The model under review builds one solid part; all positions refer to its coordinate system, in mm. Face numbers are marked on the shaded views. A direction names the side the tool comes from. Coordinates: 2 decimals unless noted, no trailing zeros. Write each loop counter-clockwise with the first axis right and the second up, starting at its lowest first coordinate (ties: lowest second). Pieces come first, ordered by that corner, then holes.
1) Add section C-C, the plane z = -109. State the section outline as (x, y) points, then the cut area to 3 significant figures.
2) For P1, Ø6, axis at x = -9, z = -30, coming from the +Y side; P2, Ø5, axis at x = 31.5, z = -21, coming from the +Y side; P3, Ø1, axis at x = 27.5, z = -31.5, coming from the -Y side; P4, Ø2.5, axis at x = -1.5, y = 12, coming from the -Z side, all flat-tipped, find the tip position at first contact; note any pin that passes through.
3) Add section D-D, the plane y = 25. State the section outline as (x, z) points.
4) Add section A-A, the plane x = -21.5. State the section outline as (y, z) points.
5) Machinability: for the marked faces 1 and 2, which of the approach directions +Z, -Z, +X, -X, +Y, -Y give a long, thin tool a straight path to every point of the face, cutting with its end or side? Answer none if there is none.
6) Add section B-B, the plane z = -127. State the section outline as (x, y) points, then the cut area to 3 significant figures.
7) For line 1 (Y direction, x = -11.5, z = -139.5); line 2 (Y direction, x = 4, z = -77); line 3 (Y direction, x = 8.5, z = -60), list the stretches that pass through material, from the lowest coordinate up.
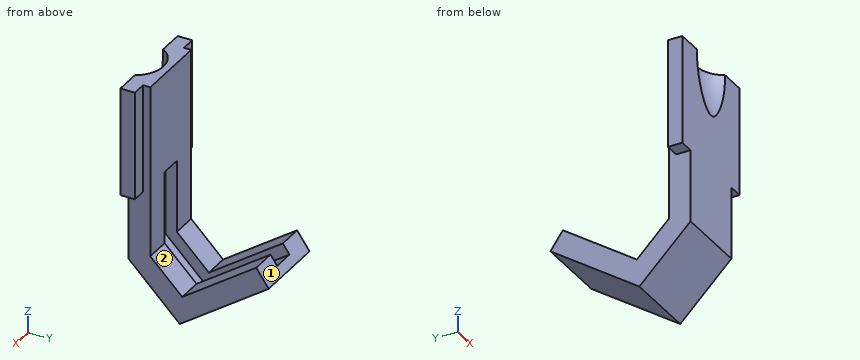
from build123d import *

# Parameters (mm, degrees)
BOSS_EXTRUDE2_DEPTH = 25
CUT_EXTRUDE1_DEPTH  = 7.5
SKETCH4_W           = 10
SKETCH4_H           = 75
BOSS_EXTRUDE3_DEPTH = 10


with BuildPart() as part:
    # Sketch2 → Boss-Extrude2 (new, symmetric)
    with BuildSketch(Plane(origin=(0, 0, 0), x_dir=(0, 0, -1), z_dir=(1, 0, 0))):
        Polygon((0, 0), (125, 0), (160.355339059, 35.355339059), (117.337106333, 96.791742381), (105.049825669, 88.188095836), (140.848741752, 37.061945188), (118.786796564, 15), (0, 15), align=None)
    extrude(amount=BOSS_EXTRUDE2_DEPTH, both=True)

    # Sketch3 → Cut-Extrude1 (cut, symmetric)
    with BuildSketch(Plane(origin=(0, 0, 0), x_dir=(0, 0, -1), z_dir=(1, 0, 0))):
        Polygon((111.603042023, 92.776707327), (151.252260316, 36.151755253), (122.100505063, 7), (68.786796564, 7), (68.786796564, 15), (118.786796564, 15), (140.848741752, 37.061945188), (105.049825669, 88.188095836), align=None)
    extrude(amount=CUT_EXTRUDE1_DEPTH, both=True, mode=Mode.SUBTRACT)

    # Sketch4 → Boss-Extrude3 (add)
    with BuildSketch(Plane(origin=(0, 0, 0), x_dir=(1, 0, 0), z_dir=(0, 1, 0))):
        with Locations((-30, 37.5)):
            Rectangle(SKETCH4_W, SKETCH4_H)
        with Locations((30, 37.5)):
            Rectangle(SKETCH4_W, SKETCH4_H)
    extrude(amount=BOSS_EXTRUDE3_DEPTH)

    # Sketch8 → Cut-Revolve5 (revolve, cut)
    with BuildSketch(Plane(origin=(0, 0, 0), x_dir=(0, 0, -1), z_dir=(1, 0, 0))):
        with BuildLine():
            Line((0, 0), (0, 10))
            ThreePointArc((0, 10), (19.364916731, 7.456883731), (37.416573868, 0))
            Line((37.416573868, 0), (0, 0))
        make_face()
    revolve(axis=Axis((0, -10, 0), (0, 0, -1)), mode=Mode.SUBTRACT)


solid = part.part
Geometry results:
1. outline: (-25, 0) - (25, 0) - (25, 15) - (7.5, 15) - (7.5, 7) - (-7.5, 7) - (-7.5, 15) - (-25, 15) - close; (-25, 82.55) - (-7.5, 82.55) - (-7.5, 90.95) - (-25, 90.95) - close; (7.5, 82.55) - (25, 82.55) - (25, 90.95) - (7.5, 90.95) - close
1. area: 924 mm2
2. P1: stops at y = 15
2. P2: stops at y = 10
2. P3: stops at y = 0
2. P4: stops at z = -138.25
3. outline: (-25, -150) - (25, -150) - (25, -128.79) - (7.5, -128.79) - (7.5, -140.1) - (-7.5, -140.1) - (-7.5, -128.79) - (-25, -128.79) - close
4. outline: (0, -125) - (35.36, -160.36) - (96.79, -117.34) - (88.19, -105.05) - (37.06, -140.85) - (15, -118.79) - (15, 0) - (0, 0) - close
5. face 1: +Z, +X, -X, +Y
5. face 2: +Z, +X, -X
6. outline: (-25, 2) - (25, 2) - (25, 23.21) - (7.5, 23.21) - (7.5, 11.9) - (-7.5, 11.9) - (-7.5, 23.21) - (-25, 23.21) - close; (-25, 56.84) - (-7.5, 56.84) - (-7.5, 70.79) - (7.5, 70.79) - (7.5, 56.84) - (25, 56.84) - (25, 82.99) - (-25, 82.99) - close
6. area: 1,990 mm2
7. line 1: y = 14.5 to 35.71, 38.99 to 65.14
7. line 2: y = 0 to 7
7. line 3: y = 0 to 15
